Can you work these out from the model? Positions are in its coordinate system, mm. A direction names the side the tool comes from. Round coordinates to 2 decimals unless told otherwise and drop trailing zeros. Loops run counter-clockwise (first coordinate to the right, second up) from the corner with the lowest first, then second, coordinate; pieces in that order, holes last. Notation, with made-up numbers: (76, 64.25) -> (128, 64.25) arc R21 cw to (128, 77.25) -> close; hole circle Ø5 at (24.5, -20.5). An arc over 180 degrees is marked (long way). Write item = value, one per line.
from build123d import *

# Parameters (mm, degrees)
BOSS_EXTRUDE1_DEPTH  = 20.5
BOSS_EXTRUDE2_START  = 5
BOSS_EXTRUDE2_DEPTH  = 5
BOSS_EXTRUDE3_DEPTH  = 5
FILLET1_R            = 2
SKETCH8_R            = 2.9
CUT_EXTRUDE4_DEPTH   = 5
FILLET1_OF_MIRROR3_R = 2
FILLET2_R            = 2.5


with BuildPart() as part:
    # Sketch1 → Boss-Extrude1 (new, symmetric)
    with BuildSketch(Plane(origin=(0, 0, 0), x_dir=(1, 0, 0), z_dir=(0, 1, 0))):
        with BuildLine():
            Line((-15.4, 0), (-17, 0))
            ThreePointArc((-17, 0), (0, 17), (17, 0))
            Line((17, 0), (15.4, 0))
            ThreePointArc((15.4, 0), (0, 15.4), (-15.4, 0))
        make_face()
    extrude(amount=BOSS_EXTRUDE1_DEPTH, both=True)

    # Sketch6 → Boss-Extrude2 (add)
    with BuildSketch(Plane(origin=(0, 20.5, 0), x_dir=(1, 0, 0), z_dir=(0, 1, 0)).offset(BOSS_EXTRUDE2_START)):
        with BuildLine():
            Line((-17, 0), (-7, 0))
            ThreePointArc((-7, 0), (0, 7), (7, 0))
            Line((7, 0), (17, 0))
            ThreePointArc((17, 0), (0, 17), (-17, 0))
        make_face()
    boss_extrude2 = extrude(amount=-BOSS_EXTRUDE2_DEPTH)

    # Mirror1: Boss-Extrude2 across plane
    add(boss_extrude2.mirror(Plane.ZX))

    # Sketch7 → Boss-Extrude3 (add, symmetric)
    with BuildSketch(Plane(origin=(0, 0, 0), x_dir=(1, 0, 0), z_dir=(0, 1, 0))):
        with BuildLine():
            Line((-17, 0), (-27, 0))
            Line((-27, 0), (-27, 5))
            Line((-27, 5), (-16.248076809, 5))
            ThreePointArc((-16.248076809, 5), (-16.810968231, 2.528111374), (-17, 0))
        make_face()
    boss_extrude3 = extrude(amount=BOSS_EXTRUDE3_DEPTH, both=True)

    # Fillet1
    fillet1_edges = [part.edges().sort_by_distance(p)[0] for p in [
        (-16.810968231, -5, -2.528111374),
        (-16.248076809, 0, -5),
        (-16.810968231, 5, -2.528111374),
    ]]
    fillet(fillet1_edges, radius=FILLET1_R)

    # Sketch8 → Cut-Extrude4 (cut, symmetric)
    with BuildSketch(Plane(origin=(0, 0, -5), x_dir=(-1, 0, 0), z_dir=(0, 0, -1))):
        with Locations((23.436686237, 0)):
            Circle(SKETCH8_R)
    cut_extrude4 = extrude(amount=CUT_EXTRUDE4_DEPTH, both=True, mode=Mode.SUBTRACT)

    # Mirror3: Boss-Extrude3, Cut-Extrude4 across plane
    add(boss_extrude3.mirror(Plane(origin=(0, 0, 0), x_dir=(0, 0, 1), z_dir=(1, 0, 0))))
    add(cut_extrude4.mirror(Plane(origin=(0, 0, 0), x_dir=(0, 0, 1), z_dir=(1, 0, 0))), mode=Mode.SUBTRACT)

    # Fillet1 of Mirror3
    fillet1_of_mirror3_edges = [part.edges().sort_by_distance(p)[0] for p in [
        (16.810968231, -5, -2.528111374),
        (16.248076809, 0, -5),
        (16.810968231, 5, -2.528111374),
    ]]
    fillet(fillet1_of_mirror3_edges, radius=FILLET1_OF_MIRROR3_R)

    # Fillet2
    fillet2_edges = [part.edges().sort_by_distance(p)[0] for p in [
        (-27, -5, -2.5),
        (-27, 5, -2.5),
        (27, 5, -2.5),
        (27, -5, -2.5),
    ]]
    fillet(fillet2_edges, radius=FILLET2_R)


solid = part.part
1. I'm going to push flat-ended pins straight in: pin 1 (3 mm diameter, centred on y = -1, z = -5.5, fed in from -X); pin 2 (3 mm diameter, centred on x = -20.5, y = -0.5, fed in from -Z); pin 3 (1.5 mm diameter, centred on x = -21, z = -2, fed in from +Y); pin 4 (5 mm diameter, centred on y = -8, z = -8.5, fed in from +X). Where does each tip first touch, or does it pass through?
Entries:
pin_1 = -27
pin_2 = -5
pin_3 = 5
pin_4 = 15.91
2. Suppose I cut it at A-A, the plane y = 0. List the corners of the cut face in (x, z) for me.
Entries:
outline = (-27, -5) -> (-26.34, -5) -> (-26.34, 0) -> (-27, 0) -> close; (-20.54, -5) -> (-17.66, -5) arc R2 cw to (-15.8, -6.26) arc R17 ccw to (15.8, -6.26) arc R2 cw to (17.66, -5) -> (20.54, -5) -> (20.54, 0) -> (15.4, 0) arc R15.4 cw to (-15.4, 0) -> (-20.54, 0) -> close; (26.34, -5) -> (27, -5) -> (27, 0) -> (26.34, 0) -> close
3. Suppose I cut it at C-C, the plane z = -11. List the corners of the cut face in (x, y) for me.
Entries:
outline = (-12.96, -25.5) -> (12.96, -25.5) -> (12.96, 25.5) -> (-12.96, 25.5) -> close; hole (-10.78, -20.5) -> (10.78, -20.5) -> (10.78, 20.5) -> (-10.78, 20.5) -> close
4. We'd pull the mould along X, two halves only. Please class faces 1 (the cylindrical face through (0.339, 0.287, -15.396)), 2 (the flat face through (0, 25.5, -9)), 3 (the cylindrical face through (0, -23, -7)), 4 (the cylindrical face through (26.248, -4.287, -2.535)): released by +X, released by -X, zero draft, split by the parting line, or undercut.
Entries:
face_1 = undercut
face_2 = zero draft
face_3 = undercut
face_4 = released by +X
5. I need wall thicknesses on line 1 (Y direction, x = 5, z = -14.25); line 2 (X direction, y = 10.5, z = -6.5); line 3 (X direction, y = 0, z = -10.5). Which ranges of each line are inside material? Lowest first, please. Write a range as [from, to].
Entries:
line_1 = [-25.5, -20.5], [20.5, 25.5]
line_2 = [-15.71, -13.96], [13.96, 15.71]
line_3 = [-13.37, -11.27], [11.27, 13.37]
6. Suppose I cut it at D-D, the plane z = -3.5. Count the separate pieces of the cut face and the enclosed holes in it, and give its area (3 significant figures).
Entries:
separate_pieces = 2
enclosed_holes = 2
area = 498 mm²
7. For faces 5 (the flat face through (0, -20.5, -8)), 6 (the flat face through (-20, 0, -5)), 7 (the cylindrical face through (-20.54, 0.13, -2.54)), which set-ups out of +Z, -Z, +X, -X, +Y, -Y let a thin tool reach every point of the face, with its end or its side?
Entries:
face_5 = +Z
face_6 = -Z, -X, +Y, -Y
face_7 = +Z, -Z
8. Suppose I cut it at B-B, the plane x = 0. List the corners of the cut face in (y, z) for me.
Entries:
outline = (-25.5, -17) -> (25.5, -17) -> (25.5, -7) -> (20.5, -7) -> (20.5, -15.4) -> (-20.5, -15.4) -> (-20.5, -7) -> (-25.5, -7) -> close
